from build123d import *

# Parameters (mm, degrees)
BOSS_EXTRUDE1_DEPTH            = 8
CHAMFER1_SIZE                  = 0.5
M3X0_5_TAPPED_HOLE1_D          = 2.5
M3X0_5_TAPPED_HOLE1_DEPTH      = 3.5
M3X0_5_TAPPED_HOLE1_TIP        = 0.751075774
F_1_8_1_8_DIAMETER_HOLE1_D     = 1.8
F_1_8_1_8_DIAMETER_HOLE1_DEPTH = 2
F_1_8_1_8_DIAMETER_HOLE1_TIP   = 0.540774557
F_1_6_1_6_DIAMETER_HOLE1_D     = 1.6
F_1_6_1_6_DIAMETER_HOLE1_DEPTH = 4.5
F_1_6_1_6_DIAMETER_HOLE1_TIP   = 0.480688495
M3X0_5_TAPPED_HOLE2_D          = 2.5
M6X1_0_TAPPED_HOLE1_D          = 6


with BuildPart() as part:
    # Sketch1 → Boss-Extrude1 (new body, symmetric)
    with BuildSketch(Plane.XY):
        with BuildLine():
            Line((-10, -0.75), (-4.381405907, -0.75))
            ThreePointArc((-4.381405907, -0.75), (1.55, -1.75), (-4.381405907, -2.75))
            Line((-4.381405907, -2.75), (-10, -2.75))
            Line((-10, -2.75), (-10, -5.75))
            Line((-10, -5.75), (10, -5.75))
            Line((10, -5.75), (10, 5.75))
            Line((10, 5.75), (-10, 5.75))
            Line((-10, 5.75), (-10, -0.75))
        make_face()
    extrude(amount=BOSS_EXTRUDE1_DEPTH, both=True)

    # Chamfer1
    chamfer1_edges = [part.edges().sort_by_distance(p)[0] for p in [
        (-10, 2.5, 8),
        (0, 5.75, -8),
        (10, 0, -8),
        (10, -5.75, 0),
        (-10, -5.75, 0),
        (-10, 5.75, 0),
        (10, 5.75, 0),
        (-10, -4.25, 8),
        (0, -5.75, 8),
        (10, 0, 8),
        (0, 5.75, 8),
        (0, -5.75, -8),
        (-10, -4.25, -8),
        (-10, 2.5, -8),
    ]]
    chamfer(chamfer1_edges, length=CHAMFER1_SIZE)

    # M3x0.5 Tapped Hole1
    with Locations(Plane.XY.offset(8)):
        with Locations((6.5, -0.95)):
            Hole(M3X0_5_TAPPED_HOLE1_D / 2, depth=M3X0_5_TAPPED_HOLE1_DEPTH)
            with Locations((0, 0, -(M3X0_5_TAPPED_HOLE1_DEPTH + M3X0_5_TAPPED_HOLE1_TIP / 2))):  # 118° drill point
                Cone(0, M3X0_5_TAPPED_HOLE1_D / 2, M3X0_5_TAPPED_HOLE1_TIP, mode=Mode.SUBTRACT)

    # Ø1.8 (1.8) Diameter Hole1
    with Locations(Plane.XY.offset(8)):
        with Locations((8, -3.75)):
            Hole(F_1_8_1_8_DIAMETER_HOLE1_D / 2, depth=F_1_8_1_8_DIAMETER_HOLE1_DEPTH)
            with Locations((0, 0, -(F_1_8_1_8_DIAMETER_HOLE1_DEPTH + F_1_8_1_8_DIAMETER_HOLE1_TIP / 2))):  # 118° drill point
                Cone(0, F_1_8_1_8_DIAMETER_HOLE1_D / 2, F_1_8_1_8_DIAMETER_HOLE1_TIP, mode=Mode.SUBTRACT)

    # Ø1.6 (1.6) Diameter Hole1
    with Locations(Plane.XY.offset(8)):
        with Locations((8, -3.75)):
            Hole(F_1_6_1_6_DIAMETER_HOLE1_D / 2, depth=F_1_6_1_6_DIAMETER_HOLE1_DEPTH)
            with Locations((0, 0, -(F_1_6_1_6_DIAMETER_HOLE1_DEPTH + F_1_6_1_6_DIAMETER_HOLE1_TIP / 2))):  # 118° drill point
                Cone(0, F_1_6_1_6_DIAMETER_HOLE1_D / 2, F_1_6_1_6_DIAMETER_HOLE1_TIP, mode=Mode.SUBTRACT)

    # M3x0.5 Tapped Hole2 (through all)
    with Locations(Plane(origin=(0, 5.75, 0), x_dir=(1, 0, 0), z_dir=(0, 1, 0))):
        with Locations((-7.5, 0)):
            Hole(M3X0_5_TAPPED_HOLE2_D / 2)

    # M6x1.0 Tapped Hole1 (through all)
    with Locations(Plane(origin=(0, 5.75, 0), x_dir=(1, 0, 0), z_dir=(0, 1, 0))):
        with Locations((6.053799896, 0)):
            Hole(M6X1_0_TAPPED_HOLE1_D / 2)


solid = part.part
CAD build for the part. Positions are in the model's coordinates, mm. A direction names the side the tool comes from. Coordinates: 2 decimals unless noted, no trailing zeros. Write each loop counter-clockwise with the first axis right and the second up, starting at its lowest first coordinate (ties: lowest second). Pieces come first, ordered by that corner, then holes. Notation, with made-up numbers: M -8.75,-20.5 L 12.25,-20.5 A20 ccw 12.25,-13.5 Z; hole C 63.25,12 d1. An arc over 180 degrees is marked long. Return JSON: item names as keys, results as strings.
Item 1: Slice it at B-B, the plane z = 0. Write the cut outline in (x, y), and give its area (3 significant figures).
Findings below:
{"outline": "M -10,-5.25 L -9.5,-5.75 L -8.75,-5.75 L -8.75,-2.75 L -10,-2.75 Z; M -10,-0.75 L -8.75,-0.75 L -8.75,5.75 L -9.5,5.75 L -10,5.25 Z; M -6.25,-5.75 L 3.05,-5.75 L 3.05,5.75 L -6.25,5.75 L -6.25,-0.75 L -4.38,-0.75 A3.05 cw long -4.38,-2.75 L -6.25,-2.75 Z; M 9.05,-5.75 L 9.5,-5.75 L 10,-5.25 L 10,5.25 L 9.5,5.75 L 9.05,5.75 Z", "area": "96.5 mm2"}
Item 2: Slice it at D-D, the plane z = 5. Write the cut outline in (x, y).
Findings below:
{"outline": "M -10,-5.25 L -9.5,-5.75 L 9.5,-5.75 L 10,-5.25 L 10,5.25 L 9.5,5.75 L -9.5,5.75 L -10,5.25 L -10,-0.75 L -4.38,-0.75 A3.05 cw long -4.38,-2.75 L -10,-2.75 Z; hole C 6.5,-0.95 d2.5; hole C 8,-3.75 d1.6"}
Item 3: Probe line 1 (Y direction, x = 8, z = 4.1); line 2 (Y direction, x = -4.75, z = -3); line 3 (X direction, y = -3.75, z = 6.85). List the from-to ranges inside material, lowest first. Write a range as from..to.
Findings below:
{"line 1": "y = -5.75..-4.55, -2.95..5.75", "line 2": "y = -5.75..-2.75, -0.75..5.75", "line 3": "x = -10..-3.8, 0.8..7.1, 8.9..10"}
Item 4: Two-plate mould, pull along Z, no slides. Class faces 1 (the flat face through (10, 0, 0)), 2 (the flat face through (-0.1, 1.2, -8)), 3 (the cylindrical face through (-6.25, 2.45, -0.05)), 4 (the cylindrical face through (-6.25, -4.27, -0.05)): +Z half, -Z half, draft (parallel to the pull), parting line (faces both ways), or undercut.
Findings below:
{"face 1": "draft", "face 2": "-Z half", "face 3": "undercut", "face 4": "undercut"}
Item 5: Slice it at C-C, the plane y = 2. Write the cut outline in (x, z), and give its area (3 significant figures).
Findings below:
{"outline": "M -10,-7.5 L -9.5,-8 L 9.5,-8 L 10,-7.5 L 10,7.5 L 9.5,8 L -9.5,8 L -10,7.5 Z; hole C -7.5,0 d2.5; hole C 6.05,0 d6", "area": "286 mm2"}
Item 6: Which spindle directions (+Z, -Z, +X, -X, +Y, -Y) get a long thin tool onto all of the face, cutting with end or side? Do faces 5 (the flat face through (-6, -2.75, 0)), 6 (the flat face through (-10, -4, 0)), 7 (the cylindrical face through (7.75, -0.9, 6.23)). Say none if no direction does.
Findings below:
{"face 5": "+Z, -Z, -X", "face 6": "+Z, -Z, -X, +Y, -Y", "face 7": "+Z"}
Item 7: Slice it at A-A, the plane x = -1.5. Write the cut outline in (y, z), and give its area (3 significant figures).
Findings below:
{"outline": "M -5.75,-7.5 L -5.25,-8 L -4.8,-8 L -4.8,8 L -5.25,8 L -5.75,7.5 Z; M 1.3,-8 L 5.25,-8 L 5.75,-7.5 L 5.75,7.5 L 5.25,8 L 1.3,8 Z", "area": "85.9 mm2"}
Item 8: Drop flat-ended pins along their axis: pin 1 Ø5.5 at (x, z) = (6.05, 0) entering from -Y; pin 2 Ø2 at (x, y) = (6.5, -0.95) entering from +Z. Give the stop position or say it passes through.
Findings below:
{"pin 1": "passes through", "pin 2": "stops at z = 4.35"}
